from build123d import *

# Parameters (mm, degrees)
SKETCH_1_R      = 2.1
EXTRUDE_1_DEPTH = 3
FILLET_1_R      = 3


with BuildPart() as part:
    # 草图1 → 凸台-拉伸1 (new body)
    with BuildSketch(Plane(origin=(0, 0, 0), x_dir=(1, 0, 0), z_dir=(0, 1, 0))):
        Polygon((-30.495345075, 10), (14.490413826, 10), (-25.409775328, -95.148540432), align=None)
        with Locations(Location((0, 0, 0), (0, 0, 270))):
            Circle(SKETCH_1_R, mode=Mode.SUBTRACT)
        with Locations(Location((-20, 0, 0), (0, 0, 270))):
            Circle(SKETCH_1_R, mode=Mode.SUBTRACT)
        with Locations(Location((-8.869515627, -23.373739379, 0), (0, 0, 270))):
            Circle(SKETCH_1_R, mode=Mode.SUBTRACT)
        with Locations(Location((-17.739031253, -46.747478758, 0), (0, 0, 270))):
            Circle(SKETCH_1_R, mode=Mode.SUBTRACT)
    extrude(amount=EXTRUDE_1_DEPTH)

    # 圆角1
    fillet_1_edges = [part.edges().sort_by_distance(p)[0] for p in [
        (-30.495345075, 1.5, -10),
        (14.490413826, 1.5, -10),
        (-25.409775328, 1.5, 95.148540432),
    ]]
    fillet(fillet_1_edges, radius=FILLET_1_R)


solid = part.part
Could you check a few things on this model? Use its own coordinates, in mm. Coordinates: 2 decimals unless noted, no trailing zeros. Order: outer loops, then holes, each group sorted by start corner. A loop starts at its lowest first (then second) coordinate and runs counter-clockwise, first axis right, second up. Notation, with made-up numbers: (-16, -33.75) -> (33, -33.75) arc R8 ccw to (33, -27.75) -> close; hole circle Ø3 at (63.25, 84). An arc over 180 degrees is marked (long way). One line per item, written item: value. Start each with the question number.
1) Imagine slicing it at D-D on z = 20. List the corners of the cut face in (x, y) for me, plus the area to 3 significant figures.
2) If I drill on L1, parallel to X at y = 0.9, z = 52; L2, parallel to X at y = 0.4, z = 43; L3, parallel to Z at x = -24.5, y = 2.1, over which ranges is the centre line in solid material (lowest first)? Write a range as [from, to].
3) Imagine slicing it at C-C on z = 0. List the corners of the cut face in (x, y) for me, plus the area to 3 significant figures.
4) Imagine slicing it at A-A on x = 0. List the corners of the cut face in (y, z) for me, plus the area to 3 significant figures.
5) We'd pull the mould along Z, two halves only. Please class faces 1 (the cylindrical face through (-18.54, 1.48, 48.69)), 2 (the flat face through (-28.194, 1.479, 37.572)), 3 (the cylindrical face through (12.589, 1.521, -8.737)): +Z half, -Z half, draft (parallel to the pull), parting line (faces both ways), or undercut.
6) Imagine slicing it at B-B on y = 1.35. List the corners of the cut face in (x, z) for me.
Answer list:
1. outline: (-29.04, 0) -> (3.11, 0) -> (3.11, 3) -> (-29.04, 3) -> close
1. area: 96.5 mm2
2. L1: x = [-27.5, -9.04]
2. L2: x = [-27.93, -5.62]
2. L3: z = [-10, 83.29]
3. outline: (-30.01, 0) -> (-22.1, 0) -> (-22.1, 3) -> (-30.01, 3) -> close; (-17.9, 0) -> (-2.1, 0) -> (-2.1, 3) -> (-17.9, 3) -> close; (2.1, 0) -> (10.7, 0) -> (10.7, 3) -> (2.1, 3) -> close
3. area: 96.9 mm2
4. outline: (0, -10) -> (3, -10) -> (3, -2.1) -> (0, -2.1) -> close; (0, 2.1) -> (3, 2.1) -> (3, 28.19) -> (0, 28.19) -> close
4. area: 102 mm2
5. face 1: undercut
5. face 2: +Z half
5. face 3: parting line
6. outline: (-30.34, -6.86) arc R3 ccw to (-27.35, -10) -> (10.14, -10) arc R3 ccw to (12.95, -5.94) -> (-20.3, 81.69) arc R3 ccw to (-26.11, 80.77) -> close; hole circle Ø4.2 at (-20, 0); hole circle Ø4.2 at (-17.74, 46.75); hole circle Ø4.2 at (-8.87, 23.37); hole circle Ø4.2 at (0, 0)
